Model file for the job. Use its own axes, mm. Face numbers are marked on the shaded views. A direction names the side the tool comes from. Coordinates: 2 decimals unless noted, no trailing zeros. Loops run counter-clockwise (first coordinate to the right, second up) from the corner with the lowest first, then second, coordinate; pieces in that order, holes last. Notation, with made-up numbers: (-27.5, 32.5) -> (1.5, 32.5) arc R25 ccw to (1.5, 54.5) -> close; hole circle Ø5 at (-33.5, 36.25). An arc over 180 degrees is marked (long way). Use one line per item in the form item = value.
```python
from build123d import *

# Parameters (mm, degrees)
F0_W      = 138.1484791636
F0_H      = 52.3216351867
F1_DEPTH  = 38.1
F2_W      = 124.6868036687
F2_H      = 5.9200678952
F3_DEPTH  = 38.1
F4_W      = 138.1484791636
F4_H      = 38.1
F5_DEPTH  = 2.54
F6_W      = 138.1484791636
F6_H      = 38.1
F7_DEPTH  = 59.69
F8_W      = 122.7258816361
F8_H      = 20.7270383835
F12_DEPTH = 33.782
F9_W      = 123.8167844713
F9_H      = 25.0906273723
F13_DEPTH = 33.782
F10_W     = 125.1115500927
F10_H     = 19.0701205283
F14_DEPTH = 33.782
F11_W     = 123.3779042959
F11_H     = 21.381651517
F15_DEPTH = 33.782


# Not quite as in the source:
# - a feature names something its author has since deleted; it is built from what else it names


with BuildPart() as f1:
    # F0 (on Front) → F1 (new body)
    with BuildSketch(Plane.XZ):
        with Locations((0.4136152565, 26.1608175933)):
            Rectangle(F0_W, F0_H)
    extrude(amount=F1_DEPTH)

    # F2 (on face) → F3 (join)
    with BuildSketch(Plane.XY.offset(52.3216351867)):
        Polygon((-61.9600676, 0), (-68.6606243253, 0), (-68.6606243253, -38.1), (-61.9600676, -38.1), (-61.9600676, -5.9200678952), align=None)
        with Locations((0.3833342344, -2.9600339476)):
            Rectangle(F2_W, F2_H)
        Polygon((69.4878548384, 0), (62.7267360687, 0), (62.7267360687, -5.9200678952), (62.7267360687, -38.1), (69.4878548384, -38.1), align=None)
    extrude(amount=F3_DEPTH)

    # F4 (on face) → F5 (join)
    with BuildSketch(Plane.XY.offset(90.4216351867)):
        with Locations((0.4136152565, -19.05)):
            Rectangle(F4_W, F4_H)
    extrude(amount=F5_DEPTH)

    # F6 (on face) → F7 (join)
    with BuildSketch(Plane.XY.offset(92.9616351867)):
        with Locations((0.4136152565, -19.05)):
            Rectangle(F6_W, F6_H)
    extrude(amount=F7_DEPTH)

    # F8 (on face) → F12 (cut)
    with BuildSketch(Plane.XZ.offset(38.1)):
        with Locations((0.1238100231, 104.7143563628)):
            Rectangle(F8_W, F8_H)
    extrude(amount=-F12_DEPTH, mode=Mode.SUBTRACT)

    # F9 (on face) → F13 (cut)
    with BuildSketch(Plane.XZ.offset(38.1)):
        with Locations((-0.694366172, 132.8049488366)):
            Rectangle(F9_W, F9_H)
    extrude(amount=-F13_DEPTH, mode=Mode.SUBTRACT)

    # F10 (on face) → F14 (cut)
    with BuildSketch(Plane.XZ.offset(38.1)):
        with Locations((0.7500052452, 37.6429138705)):
            Rectangle(F10_W, F10_H)
    extrude(amount=-F14_DEPTH, mode=Mode.SUBTRACT)

    # F11 (on face) → F15 (cut)
    with BuildSketch(Plane.XZ.offset(38.1)):
        with Locations((1.0389462113, 14.81655729)):
            Rectangle(F11_W, F11_H)
    extrude(amount=-F15_DEPTH, mode=Mode.SUBTRACT)


solid = f1.part
```
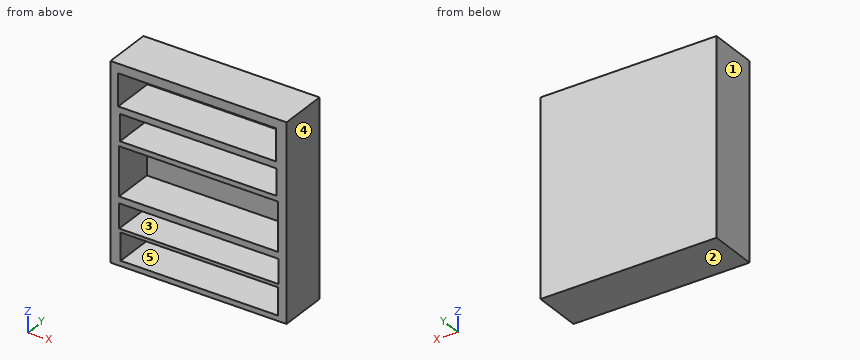
Q1. Band-saw the part on D-D, the plane z = 83. Write the cut outline in (x, y).
Result:
outline = (-68.66, -38.1) -> (-61.96, -38.1) -> (-61.96, -5.92) -> (62.73, -5.92) -> (62.73, -38.1) -> (69.49, -38.1) -> (69.49, 0) -> (-68.66, 0) -> close
Q2. Band-saw the part on A-A, the plane y = -11. Write the cut outline in (x, z).
Result:
outline = (-68.66, 0) -> (69.49, 0) -> (69.49, 152.65) -> (-68.66, 152.65) -> close; hole (-62.6, 120.26) -> (61.21, 120.26) -> (61.21, 145.35) -> (-62.6, 145.35) -> close; hole (-61.96, 52.32) -> (62.73, 52.32) -> (62.73, 90.42) -> (-61.96, 90.42) -> close; hole (-61.81, 28.11) -> (63.31, 28.11) -> (63.31, 47.18) -> (-61.81, 47.18) -> close; hole (-61.24, 94.35) -> (61.49, 94.35) -> (61.49, 115.08) -> (-61.24, 115.08) -> close; hole (-60.65, 4.13) -> (62.73, 4.13) -> (62.73, 25.51) -> (-60.65, 25.51) -> close
Q3. Band-saw the part on C-C, the plane x = -22. Write the cut outline in (y, z), and give its area (3 significant figures).
Result:
outline = (-38.1, 0) -> (0, 0) -> (0, 152.65) -> (-38.1, 152.65) -> (-38.1, 145.35) -> (-4.32, 145.35) -> (-4.32, 120.26) -> (-38.1, 120.26) -> (-38.1, 115.08) -> (-4.32, 115.08) -> (-4.32, 94.35) -> (-38.1, 94.35) -> (-38.1, 90.42) -> (-5.92, 90.42) -> (-5.92, 52.32) -> (-38.1, 52.32) -> (-38.1, 47.18) -> (-4.32, 47.18) -> (-4.32, 28.11) -> (-38.1, 28.11) -> (-38.1, 25.51) -> (-4.32, 25.51) -> (-4.32, 4.13) -> (-38.1, 4.13) -> close
area = 1,680 mm2
Q4. Pin check, flat tips, straight feed: pin 1 Ø1 at (x, z) = (10.5, 108) entering from +Y; pin 2 Ø19 at (x, z) = (24.5, 76) entering from -Y; pin 3 Ø15.5 at (x, z) = (-14.5, 38) entering from -Y. Stop position of each tip, or through.
Result:
pin_1 = 0
pin_2 = -5.92
pin_3 = -4.32
Q5. Which spindle directions (+Z, -Z, +X, -X, +Y, -Y) get a long thin tool onto all of the face, cutting with end or side? Do the marked faces 4 and 5. Say none if no direction does.
Result:
face_4 = +Z, -Z, +X, +Y, -Y
face_5 = -Y
Q6. Wall check: line 1 along Z through (x, y) = (-15, -26.5); line 2 along Z through (x, y) = (-61, -26.5); line 3 along X through (y, z) = (-23, 30). Give the ranges that are in metal, low to high.
Result:
line_1 = 0 to 4.13, 25.51 to 28.11, 47.18 to 52.32, 90.42 to 94.35, 115.08 to 120.26, 145.35 to 152.65
line_2 = 0 to 28.11, 47.18 to 52.32, 90.42 to 94.35, 115.08 to 120.26, 145.35 to 152.65
line_3 = -68.66 to -61.81, 63.31 to 69.49
Q7. Mould opens along X. For the marked faces 1, 2 and 3 say: released by +X, released by -X, zero draft, split by the parting line, or undercut.
Result:
face_1 = released by -X
face_2 = zero draft
face_3 = undercut
Q8. Band-saw the part on B-B, the plane z = 104. Write the cut outline in (x, y).
Result:
outline = (-68.66, -38.1) -> (-61.24, -38.1) -> (-61.24, -4.32) -> (61.49, -4.32) -> (61.49, -38.1) -> (69.49, -38.1) -> (69.49, 0) -> (-68.66, 0) -> close
